from build123d import *

# Parameters (mm, degrees)
F0_R     = 57.21436
F1_DEPTH = 25.4
F2_R     = 46.159754
F3_DEPTH = 25.4
F4_W     = 13.088044
F4_H     = 22.873998
F5_DEPTH = 25.4


with BuildPart() as f1:
    # F0 (on Top) → F1 (new body)
    with BuildSketch(Plane.XY):
        Circle(F0_R)
    extrude(amount=F1_DEPTH)

    # F2 (on Top) → F3 (cut)
    with BuildSketch(Plane.XY):
        Circle(F2_R)
    extrude(amount=F3_DEPTH, mode=Mode.SUBTRACT)

    # F4 (on Top) → F5 (cut)
    with BuildSketch(Plane.XY):
        with Locations((0, 182.986438)):
            Rectangle(F4_W, F4_H)
    extrude(amount=F5_DEPTH, mode=Mode.SUBTRACT)


solid = f1.part
Can you work these out from the model? Positions are in its coordinate system, mm. Round coordinates to 2 decimals unless told otherwise and drop trailing zeros. Order: outer loops, then holes, each group sorted by start corner. A loop starts at its lowest first (then second) coordinate and runs counter-clockwise, first axis right, second up. Notation, with made-up numbers: (-24, 1) - (-7, 1) arc R23 ccw to (-7, 39) - close; hole circle Ø6 at (6.5, -3). An arc over 180 degrees is marked (long way). Answer in a Markdown table with one row per item.
(1) Suppose I cut it at A-A, the plane x = 0. Please give me the cut outline in (y, z).
From the geometry:
| item | result |
|---|---|
| outline | (-57.21, 0) - (-46.16, 0) - (-46.16, 25.4) - (-57.21, 25.4) - close; (46.16, 0) - (57.21, 0) - (57.21, 25.4) - (46.16, 25.4) - close |
(2) If we mould it in two halves opening along X, with no side actions, what happens to faces 1 (the face through (4, 47, 0)), 2 (the face through (26.4, -50.76, 12.52)), 3 (the face through (44.028, 13.865, 12.522))? For each: released by +X, released by -X, zero draft, split by the parting line, or undercut.
From the geometry:
| item | result |
|---|---|
| face 1 | zero draft |
| face 2 | split by the parting line |
| face 3 | undercut |
(3) Please list where these lines run through material, in increasing order: L1, parallel to Y at x = 0, z = 19; L2, parallel to X at y = 31.5, z = 12.5; L3, parallel to X at y = 40.5, z = 4.75. Write a range as from..to.
From the geometry:
| item | result |
|---|---|
| L1 | y = -57.21..-46.16, 46.16..57.21 |
| L2 | x = -47.76..-33.74, 33.74..47.76 |
| L3 | x = -40.41..-22.15, 22.15..40.41 |
(4) For P1, Ø1.5, axis at y = -45, z = 22, coming from the +X side; P2, Ø2, axis at x = -8.5, z = 7.5, coming from the -Y side; P3, Ø3, axis at x = -34.5, z = 19.5, coming from the -Y side, each with a flat end and sliding along its axis, tell me the tip position at first contact or that it passes through.
From the geometry:
| item | result |
|---|---|
| P1 | stops at x = 36.27 |
| P2 | stops at y = -56.72 |
| P3 | stops at y = -46.74 |
(5) Suppose I cut it at C-C, the plane z = 9.25. Please give me the cut outline in (x, y).
From the geometry:
| item | result |
|---|---|
| outline | circle Ø114.43 at (0, 0); hole circle Ø92.32 at (0, 0) |
